```python
from build123d import *

# Parameters (mm, degrees)
SKETCH_1_W             = 28.4
SKETCH_1_H             = 13.3
EXTRUDE_1_DEPTH        = 1
SKETCH_2_R             = 1.25
CUT_EXTRUDE_1_DEPTH    = 2
EXTRUDE_START          = -1
SKETCH_3_W             = 15.5
SKETCH_3_H             = 12
EXTRUDE_2_DEPTH        = 7
SKETCH_4_R             = 0.75
CUT_EXTRUDE_2_DEPTH    = 2
PATTERN_LINEAR_1_COUNT = 3
PATTERN_LINEAR_1_PITCH = 2.54


with BuildPart() as part:
    # 草图1 → 凸台-拉伸1 (new body)
    with BuildSketch(Plane(origin=(0, 0, 0), x_dir=(1, 0, 0), z_dir=(0, 1, 0))):
        Rectangle(SKETCH_1_W, SKETCH_1_H)
    extrude(amount=EXTRUDE_1_DEPTH)

    # 草图2 → 切除-拉伸1 (cut, through all)
    with BuildSketch(Plane(origin=(0, 1, 0), x_dir=(1, 0, 0), z_dir=(0, 1, 0))):
        with Locations((6.7, 0.35)):
            Circle(SKETCH_2_R)
    extrude(amount=-CUT_EXTRUDE_1_DEPTH, mode=Mode.SUBTRACT)

    # 草图3 → 凸台-拉伸2 (add)
    with BuildSketch(Plane(origin=(0, 1, 0), x_dir=(1, 0, 0), z_dir=(0, 1, 0)).offset(EXTRUDE_START)):
        with Locations((-6.45, 0)):
            Rectangle(SKETCH_3_W, SKETCH_3_H)
    extrude(amount=EXTRUDE_2_DEPTH)

    # 草图4 → 切除-拉伸2 (cut, through all)
    with BuildSketch(Plane(origin=(0, 1, 0), x_dir=(1, 0, 0), z_dir=(0, 1, 0))):
        with Locations((12.765289475, 3.091279596)):
            Circle(SKETCH_4_R)
    cut_extrude_2 = extrude(amount=-CUT_EXTRUDE_2_DEPTH, mode=Mode.SUBTRACT)

    # 阵列(线性)1: 切除-拉伸2 ×3
    with Locations(*[(0, 0, i * PATTERN_LINEAR_1_PITCH) for i in range(1, PATTERN_LINEAR_1_COUNT)]):
        add(cut_extrude_2, mode=Mode.SUBTRACT)


solid = part.part
```
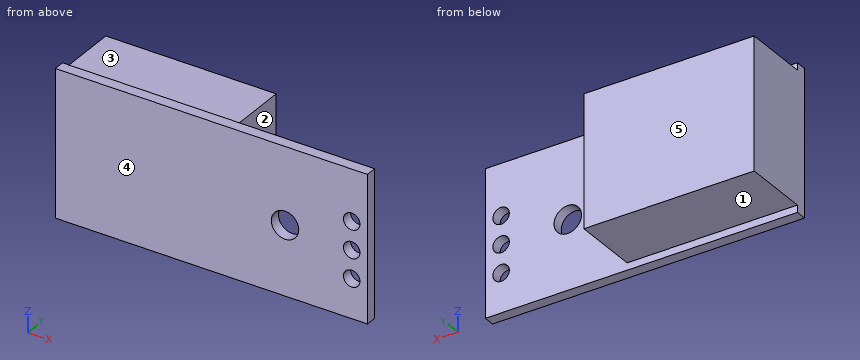
Could you check a few things on this model? Use its own coordinates, in mm. Face numbers are marked on the shaded views. A direction names the side the tool comes from. Coordinates: 2 decimals unless noted, no trailing zeros. Write each loop counter-clockwise with the first axis right and the second up, starting at its lowest first coordinate (ties: lowest second). Pieces come first, ordered by that corner, then holes. Notation, with made-up numbers: M 85.25,7 L 111.25,7 A20 ccw 111.25,15 Z; hole C 45.5,25 d4. An arc over 180 degrees is marked long. Answer as CSV lines item,"result". Start each with the question number.
1) For P1, Ø1.2, axis at x = 12.77, z = 1.99, coming from the -Y side; P2, Ø3, axis at y = 4.5, z = 2.5, coming from the +X side, each with a flat end and sliding along its axis, tell me the tip position at first contact or that it passes through.
2) I want a section at B-B, the plane z = 3. Please give me the cut outline in (x, y).
3) I want a section at C-C, the plane y = 2. Please give me the cut outline in (x, z), and give its area (3 significant figures).
4) For the marked faces 1, 2, 3, 4 and 5, which set-ups out of +Z, -Z, +X, -X, +Y, -Y let a thin tool reach every point of the face, with its end or its side?
5) Please list where these lines run through material, in increasing order: line 1 (Z direction, x = 6.7, y = 0.7); line 2 (Z direction, x = -9.5, y = 3.25); line 3 (X direction, y = 1.5, z = -4). Write a range as from..to.
6) I want a section at A-A, the plane x = 6.7. Please give me the cut outline in (y, z), and give its area (3 significant figures).
7) I want a section at D-D, the plane x = 3.5. Please give me the cut outline in (y, z).
Data:
1,P1,"passes through"
1,P2,"stops at x = 1.3"
2,outline,"M -14.2,0 L 14.2,0 L 14.2,1 L 1.3,1 L 1.3,7 L -14.2,7 Z"
3,outline,"M -14.2,-6 L 1.3,-6 L 1.3,6 L -14.2,6 Z"
3,area,"186 mm^2"
4,face 1,"-Z, +X, -X, +Y"
4,face 2,"+Z, -Z, +X, +Y"
4,face 3,"+Z, +X, -X, +Y"
4,face 4,"+Z, -Z, +X, -X, -Y"
4,face 5,"+Z, -Z, +X, -X, +Y"
5,line 1,"z = -6.65..-1.6, 0.9..6.65"
5,line 2,"z = -6..6"
5,line 3,"x = -14.2..1.3"
6,outline,"M 0,-6.65 L 1,-6.65 L 1,-1.6 L 0,-1.6 Z; M 0,0.9 L 1,0.9 L 1,6.65 L 0,6.65 Z"
6,area,"10.8 mm^2"
7,outline,"M 0,-6.65 L 1,-6.65 L 1,6.65 L 0,6.65 Z"
